For this review, take the finished solid that the model builds, in its own axes (mm). Face numbers are marked on the shaded views. A direction names the side the tool comes from. Give positions to 0.01 mm unless a question says otherwise; leave off trailing zeros. Loops run counter-clockwise (first coordinate to the right, second up) from the corner with the lowest first, then second, coordinate; pieces in that order, holes last. Notation, with made-up numbers: M 10.25,89 L 57.25,89 A14 cw 57.25,105 Z; hole C 15,-11.5 d8. An arc over 180 degrees is marked long. Use CSV: the item, a comma, the result in double quotes. Start each with the question number.
1. To check wall thickness, follow line 1 (Y direction, x = -14.75, z = 5.5); line 2 (Z direction, x = -14, y = 18.5); line 3 (Z direction, x = -16, y = 24.25). State the ranges of each line that lie inside material, in increasing order. Write a range as [from, to].
2. Take a section at D-D, the plane z = 2.25. Write out the cut boundary in (x, y).
3. Insertion check: P1, Ø1.5, axis at x = -15.5, y = 19, coming from the +Z side. The pin has a flat end and moves straight along its axis. Give the tip position at first contact, or say it passes through.
4. Take a section at A-A, the plane z = 6.75. Write out the cut boundary in (x, y), and give its area (3 significant figures).
5. Tool access review of the marked faces 4 and 5: name each direction out of +Z, -Z, +X, -X, +Y, -Y from which nothing blocks a thin tool from reaching the whole face with its end or side.
6. Take a section at B-B, the plane y = 23.5. Write out the cut boundary in (x, z).
7. Take a section at C-C, the plane x = -12.5. Write out the cut boundary in (y, z), and give its area (3 significant figures).
8. The part is to be moulded in two halves that separate along Y. For the marked faces 1, 2 and 3, say which applies: pulls with the +Y half, pulls with the -Y half, needs draft (parallel to the pull), parting line crosses it, or undercut.
Autodesk Inventor part; units mm, degrees
ref_plane "YZ Plane" through (0, 0, 0) normal (1, 0, 0) x (0, 1, 0)
ref_plane "XZ Plane" through (0, 0, 0) normal (0, 1, 0) x (-1, 0, 0)
ref_plane "XY Plane" through (0, 0, 0) normal (0, 0, 1) x (1, 0, 0)
sketch "Sketch1" plane through (0, 0, 0) normal (0, 0, 1) x (1, 0, 0)
  line L0 (-19.7239, 24.3858) -> (-9.7239, 24.3858)
  line L1 (-9.7239, 24.3858) -> (-9.7239, 14.3858)
  line L2 (-9.7239, 14.3858) -> (-19.7239, 14.3858)
  line L3 (-19.7239, 14.3858) -> (-19.7239, 24.3858)
  line L4 (-19.7239, 24.3858) -> (-9.7239, 14.3858) construction
  line L5 (-9.7239, 24.3858) -> (-19.7239, 14.3858) construction
  line L6 (-7.848, 12.2173) -> (-10.7345, 12.2561)
  line L7 (-7.848, 12.2173) -> (-12.5422, 20.6065)
  arc A0 (-12.5422, 20.6065) -> (-16.9056, 18.165) centre (-14.7239, 19.3858) ccw
  line L8 (-16.9056, 18.165) -> (-10.8018, 7.2566)
  line L9 (-10.7345, 12.2561) -> (-10.8018, 7.2566)
  circle A1 centre (-14.7239, 19.3858) radius 1.5
  circle A2 centre (-14.7239, 19.3858) radius 1.5
  line L10 (-68.8088, 12.3105) -> (-68.8088, 17.3105)
  arc A3 (-68.8088, 17.3105) -> (-78.8088, 17.3105) centre (-73.8088, 17.3105) ccw
  line L11 (-78.8088, 17.3105) -> (-78.8088, -37.6895)
  line L12 (-78.8088, -37.6895) -> (-33.8088, -37.6895)
  line L13 (-33.8088, -37.6895) -> (-28.8088, -32.6895)
  line L14 (-28.8088, -32.6895) -> (-73.8088, -32.6895)
  line L15 (-73.8088, -32.6895) -> (-73.8088, 7.3105)
  line L16 (-73.8088, 7.3105) -> (-18.8088, 7.3105)
  line L17 (-18.8088, 7.3105) -> (-12.5588, 18.1358)
  arc A4 (-12.5588, 18.1358) -> (-16.8889, 20.6358) centre (-14.7239, 19.3858) ccw
  line L18 (-16.8889, 20.6358) -> (-21.6956, 12.3105)
  line L19 (-21.6956, 12.3105) -> (-68.8088, 12.3105)
  circle A5 centre (-73.8088, 17.3105) radius 2.5
  dimension "d0" = 10
  dimension "d1" = 10
extrude "Extrusion1" add sketch "Sketch1" along normal blind 13 contours L0 L1 L7 A0 L18 L3 | L18 A0 L8 L2 L3 | L1 L2 L17 A4 L7 | A0 A4 L17 L2 L8 | A1
fillet "Fillet1" radius 2 4 edges at (-9.7239, 24.3858, 6.5) (-9.7239, 14.3858, 6.5) (-19.7239, 24.3858, 6.5) (-19.7239, 14.3858, 6.5)
sketch "Sketch2" plane through (0, 0, 13) normal (0, 0, 1) x (1, 0, 0)
  circle A0 centre (-14.7239, 19.3858) radius 1.5
  point P0 (0, 0)
extrude "Extrusion2" cut sketch "Sketch2" against normal blind 10
sketch "Sketch3" plane through (-17.7239, 24.3858, 0) normal (0, 1, 0) x (1, 0, 0)
  line L0 (0, -13) -> (0, 0)
  line L1 (6, -13) -> (0, -13)
  line L2 (6, 0) -> (6, -13)
  line L3 (6, 0) -> (0, 0)
  line L4 (0, -13) -> (0, 0)
  line L5 (0, -6.5) -> (6, -6.5)
  line L6 (6, 0) -> (6, -13)
  circle A0 centre (3, -6.5) radius 2.5
  point P0 (17.7239, 0)
  dimension "d7" = 5
extrude "Extrusion3" cut sketch "Sketch3" against normal blind 2 contours A0 L5 | L5 A0
properties part number "Claw Connector New"
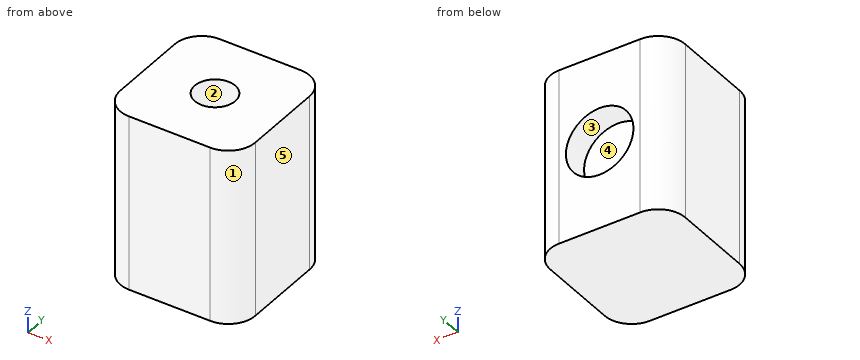
Result set:
1,line 1,"[14.39, 17.89], [20.89, 22.39]"
1,line 2,"[0, 3]"
1,line 3,"[0, 4.35], [8.65, 13]"
2,outline,"M -19.72,16.39 A2 ccw -17.72,14.39 L -11.72,14.39 A2 ccw -9.72,16.39 L -9.72,22.39 A2 ccw -11.72,24.39 L -17.72,24.39 A2 ccw -19.72,22.39 Z"
3,P1,"z = 13"
4,outline,"M -19.72,16.39 A2 ccw -17.72,14.39 L -11.72,14.39 A2 ccw -9.72,16.39 L -9.72,22.39 A2 ccw -11.72,24.39 L -12.24,24.39 L -12.24,22.39 L -17.21,22.39 L -17.21,24.39 L -17.72,24.39 A2 ccw -19.72,22.39 Z; hole C -14.72,19.39 d3"
4,area,"79.5 mm2"
5,face 4,"+Y"
5,face 5,"+Z, -Z, +X, +Y, -Y"
6,outline,"M -19.38,0 L -10.06,0 L -10.06,13 L -19.38,13 Z; hole C -14.72,6.5 d5"
7,outline,"M 14.39,0 L 24.39,0 L 24.39,5.36 L 22.39,5.36 L 22.39,7.64 L 24.39,7.64 L 24.39,13 L 14.39,13 Z"
7,area,"125 mm2"
8,face 1,"pulls with the -Y half"
8,face 2,"undercut"
8,face 3,"needs draft"
